from build123d import *

# Parameters (mm, degrees)
SKETCH_R     = 1.675
SKETCH_W     = 23
SKETCH_H     = 32
PAD_DEPTH    = 2
SKETCH001_W  = 24
SKETCH001_H  = 33.5
POCKET_DEPTH = 0.8


with BuildPart() as part:
    # Sketch → Pad (new body)
    with BuildSketch(Plane.XY):
        with BuildLine():
            ThreePointArc((-25.35, 50), (-27.471328, 49.121313), (-28.35, 46.999979))
            Line((-28.35, 46.999979), (-28.35, 43.499979))
            ThreePointArc((-28.35, 43.499979), (-27.47132, 41.378659), (-25.35, 40.499979))
            Line((-25.35, 40.499979), (-20.5, 40.499979))
            ThreePointArc((-17.5, 37.499979), (-18.37868, 39.6213), (-20.5, 40.499979))
            Line((-17.5, 37.499979), (-17.5, 0))
            Line((-17.5, 0), (17.5, 0))
            Line((17.5, 37.499979), (17.5, 0))
            ThreePointArc((20.5, 40.499979), (18.37868, 39.6213), (17.5, 37.499979))
            Line((25.35, 40.499979), (20.5, 40.499979))
            ThreePointArc((25.35, 40.499979), (27.47132, 41.378659), (28.35, 43.499979))
            Line((28.35, 43.499979), (28.35, 46.999979))
            ThreePointArc((28.35, 46.999979), (27.471328, 49.121313), (25.35, 50))
            Line((-25.35, 50), (25.35, 50))
        make_face()
        with Locations((-25.35, 47)):
            Circle(SKETCH_R, mode=Mode.SUBTRACT)
        with Locations((25.35, 47)):
            Circle(SKETCH_R, mode=Mode.SUBTRACT)
        with Locations((0, 23)):
            Rectangle(SKETCH_W, SKETCH_H, mode=Mode.SUBTRACT)
    extrude(amount=PAD_DEPTH)

    # Sketch001 → Pocket (cut)
    with BuildSketch(Plane.XY.offset(2)):
        with Locations((0, 23)):
            Rectangle(SKETCH001_W, SKETCH001_H)
    extrude(amount=-POCKET_DEPTH, mode=Mode.SUBTRACT)


solid = part.part
Source: CAD feature listing. Evaluate the final solid. Frame: model axes, mm. A direction names the side the tool comes from. Give positions to 0.01 mm unless a question says otherwise; leave off trailing zeros. Write each loop counter-clockwise with the first axis right and the second up, starting at its lowest first coordinate (ties: lowest second). Pieces come first, ordered by that corner, then holes. Notation, with made-up numbers: (79, 75) -> (121, 75) arc R20 cw to (121, 107) -> close; hole circle Ø5 at (65.5, 44.5). An arc over 180 degrees is marked (long way). Write item = value, one per line.
Q1. Cut plane B-B on y = 25.5. Return loops of the section in (x, z).
Here are the results:
outline = (-17.5, 0) -> (-11.5, 0) -> (-11.5, 1.2) -> (-12, 1.2) -> (-12, 2) -> (-17.5, 2) -> close; (11.5, 0) -> (17.5, 0) -> (17.5, 2) -> (12, 2) -> (12, 1.2) -> (11.5, 1.2) -> close
Q2. First-contact query: pin 1 (1 mm diameter, centred on y = 16.5, z = 1, fed in from -X); pin 2 (2 mm diameter, centred on x = 25.35, y = 47, fed in from +Z); pin 3 (1 mm diameter, centred on x = -21.5, z = 0.5, fed in from -Y). Flat tips, straight axial feed; report the tip coordinate or a pass-through.
Here are the results:
pin_1 = -17.5
pin_2 = through
pin_3 = 40.5
Q3. Reachability of faces 1 (the face through (-17.5, 19, 1)), 2 (the face through (28.35, 45, 1)), 3 (the face through (11.5, 23, 1)), 4 (the face through (23, 40.5, 1)) from +Z, -Z, +X, -X, +Y, -Y: full face, straight path, thin tool, end or side. Return the list, or none.
Here are the results:
face_1 = +Z, -Z, -X, -Y
face_2 = +Z, -Z, +X, +Y, -Y
face_3 = +Z, -Z
face_4 = +Z, -Z, +X, -Y
Q4. Cut plane C-C on z = 1.7. Return loops of the section in (x, y) (3 decimals), then the cut area to 3 significant figures.
Here are the results:
outline = (-28.35, 43.5) arc R3 ccw to (-25.35, 40.5) -> (-20.5, 40.5) arc R3 cw to (-17.5, 37.5) -> (-17.5, 0) -> (17.5, 0) -> (17.5, 37.5) arc R3 cw to (20.5, 40.5) -> (25.35, 40.5) arc R3 ccw to (28.35, 43.5) -> (28.35, 47) arc R3 ccw to (25.35, 50) -> (-25.35, 50) arc R3 ccw to (-28.35, 47) -> close; hole circle Ø3.35 at (-25.35, 47); hole (-12, 6.25) -> (12, 6.25) -> (12, 39.75) -> (-12, 39.75) -> close; hole circle Ø3.35 at (25.35, 47)
area = 1,130 mm²
Q5. Line query: line 1 (X direction, y = 25, z = 0.8); line 2 (Y direction, x = -25.35, z = 1.5) (3 decimals); line 3 (Y direction, x = 11, z = 1.45). Output: solid intervals per line, ascending. Write a range as from..to.
Here are the results:
line_1 = -17.5..-11.5, 11.5..17.5
line_2 = 40.5..45.325, 48.675..50
line_3 = 0..6.25, 39.75..50
Q6. Cut plane A-A on x = 10.5. Return loops of the section in (y, z).
Here are the results:
outline = (0, 0) -> (7, 0) -> (7, 1.2) -> (6.25, 1.2) -> (6.25, 2) -> (0, 2) -> close; (39, 0) -> (50, 0) -> (50, 2) -> (39.75, 2) -> (39.75, 1.2) -> (39, 1.2) -> close
Q7. Mould query, pull axis Y, two halves, no side actions, for faces 5 (the face through (18.4, 39.64, 0.99)), 6 (the face through (17.5, 19, 1)), 7 (the face through (0, 39, 1)). Classes: +Y half, -Y half, draft (parallel to the pull), parting line (faces both ways), or undercut.
Here are the results:
face_5 = -Y half
face_6 = draft
face_7 = undercut
